Check sheet for the modelled part. Datum: model origin and axes. Units: mm. Face numbers are marked on the shaded views. Round coordinates to 2 decimals unless told otherwise and drop trailing zeros. Order: outer loops, then holes, each group sorted by start corner. A loop starts at its lowest first (then second) coordinate and runs counter-clockwise, first axis right, second up. Notation, with made-up numbers: (30.25, 41) -> (88.25, 41) arc R15 cw to (88.25, 68) -> close; hole circle Ø2 at (-22.5, 26). An arc over 180 degrees is marked (long way). Answer in a Markdown table with one row per item.
```python
from build123d import *

# Parameters (mm, degrees)
ESQUISSE1_W             = 24
ESQUISSE1_H             = 38
ESQUISSE1_W_2           = 10
ESQUISSE1_H_2           = 29.5
SHAPE_DEPTH             = 1.5
ESQUISSE2_R             = 1.2
VISHOLES_DEPTH          = 1.5
ESQUISSE3_R             = 1.8
LOCKERS_DEPTH           = 2
ESQUISSE4_R             = 2.2
SCREWHATREMOVER_DEPTH   = 0.5
ESQUISSE6_W             = 24
ESQUISSE6_H             = 14.5
RALLONGE_DEPTH          = 1.5
ESQUISSE7_W             = 24
ESQUISSE7_H             = 1.5
BOSS_EXTRU_2_DEPTH      = 8.5
ESQUISSE8_R             = 1.2
ENL_V_MAT_EXTRU_1_DEPTH = 10
ESQUISSE9_R             = 1.5
BOSS_EXTRU_3_DEPTH      = 5
NERVURE11_REACH         = 48.457
ESQUISSE12_WALL_W       = 106.934753954
ESQUISSE12_WALL_H       = 1


with BuildPart() as part:
    # Esquisse1 → Shape (new body)
    with BuildSketch(Plane(origin=(0, 0, 0), x_dir=(1, 0, 0), z_dir=(0, 1, 0))):
        Rectangle(ESQUISSE1_W, ESQUISSE1_H)
        with Locations((0, 2.75)):
            Rectangle(ESQUISSE1_W_2, ESQUISSE1_H_2, mode=Mode.SUBTRACT)
    extrude(amount=SHAPE_DEPTH)

    # Esquisse2 → VisHoles (cut)
    with BuildSketch(Plane(origin=(0, 1.5, 0), x_dir=(1, 0, 0), z_dir=(0, 1, 0))):
        with Locations(Location((10, -9, 0), (0, 0, 270))):
            Circle(ESQUISSE2_R)
    visholes = extrude(amount=-VISHOLES_DEPTH, mode=Mode.SUBTRACT)

    # Esquisse3 → Lockers (add)
    with BuildSketch(Plane(origin=(0, 1.5, 0), x_dir=(1, 0, 0), z_dir=(0, 1, 0))):
        with Locations(Location((10, 11, 0), (0, 0, 90))):
            Circle(ESQUISSE3_R)
    lockers = extrude(amount=LOCKERS_DEPTH)

    # Esquisse4 → ScrewHatRemover (cut)
    with BuildSketch(Plane(origin=(0, 0, 0), x_dir=(1, 0, 0), z_dir=(0, 1, 0))):
        with Locations((10, -9)):
            Circle(ESQUISSE4_R)
    screwhatremover = extrude(amount=SCREWHATREMOVER_DEPTH, mode=Mode.SUBTRACT)

    # Symétrie1: VisHoles, Lockers, ScrewHatRemover across plane
    add(visholes.mirror(Plane(origin=(0, 0, 0), x_dir=(0, 0, 1), z_dir=(1, 0, 0))), mode=Mode.SUBTRACT)
    add(lockers.mirror(Plane(origin=(0, 0, 0), x_dir=(0, 0, 1), z_dir=(1, 0, 0))))
    add(screwhatremover.mirror(Plane(origin=(0, 0, 0), x_dir=(0, 0, 1), z_dir=(1, 0, 0))), mode=Mode.SUBTRACT)

    # Esquisse6 → Rallonge (add)
    with BuildSketch(Plane.XZ):
        with Locations((0, 26.25)):
            Rectangle(ESQUISSE6_W, ESQUISSE6_H)
    extrude(amount=-RALLONGE_DEPTH)

    # Esquisse7 → Boss.-Extru.2 (add)
    with BuildSketch(Plane(origin=(0, 1.5, 0), x_dir=(1, 0, 0), z_dir=(0, 1, 0))):
        with Locations((0, -32.75)):
            Rectangle(ESQUISSE7_W, ESQUISSE7_H)
    extrude(amount=BOSS_EXTRU_2_DEPTH)

    # Esquisse8 → Enlèv. mat.-Extru.1 (cut)
    with BuildSketch(Plane.XY.offset(33.5)):
        with Locations((0, 5)):
            Circle(ESQUISSE8_R)
    extrude(amount=-ENL_V_MAT_EXTRU_1_DEPTH, mode=Mode.SUBTRACT)

    # Esquisse9 → Boss.-Extru.3 (add)
    with BuildSketch(Plane.XY.offset(33.5)):
        with Locations((5, 5)):
            Circle(ESQUISSE9_R)
        with Locations((-5, 5)):
            Circle(ESQUISSE9_R)
    extrude(amount=BOSS_EXTRU_3_DEPTH)

    # Esquisse12 wall → Nervure11 (add, up to next)
    with BuildSketch(Plane(origin=(-12, 5.75, 27.75), x_dir=(0, -0.707106781187, -0.707106781187), z_dir=(0, -0.707106781187, 0.707106781187)), mode=Mode.PRIVATE) as nervure11_sk1:
        with Locations((0, 0.5)):
            Rectangle(ESQUISSE12_WALL_W, ESQUISSE12_WALL_H)
    nervure11_tool1 = extrude(nervure11_sk1.sketch, amount=NERVURE11_REACH, mode=Mode.PRIVATE) - part.part
    nervure11 = nervure11_tool1.solids().sort_by_distance((-12, 5.75, 27.75))[0]
    add(nervure11)

    # Symétrie2: Nervure11 across plane
    add(nervure11.mirror(Plane(origin=(0, 0, 0), x_dir=(0, 0, 1), z_dir=(1, 0, 0))))


solid = part.part
```
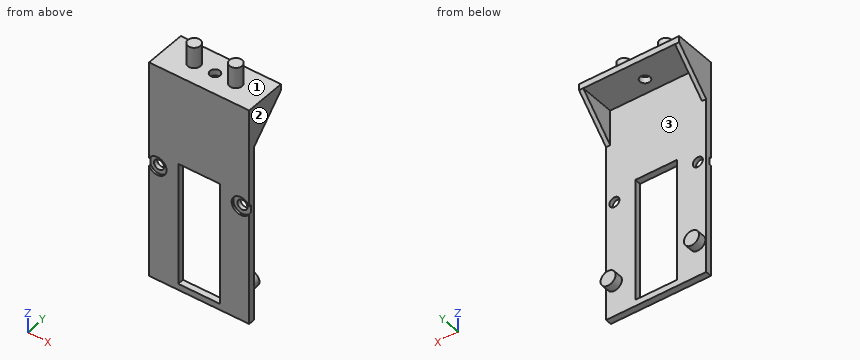
(1) Scan lines: probe 1 along X at (y, z) = (1.05, 9); probe 2 along Z at (x, y) = (-4.75, 0.5); probe 3 along Y at (x, z) = (0, 32.95). Record each from-to range of solid material in increasing order. Write a range as from..to.
Solutions:
| item | result |
|---|---|
| probe 1 | -12..-11.2, -8.8..-5, 5..8.8, 11.2..12 |
| probe 2 | -19..-17.5, 12..33.5 |
| probe 3 | 0..3.8, 6.2..10 |
(2) Section check A-A on x = -2.75. Record the boundary of the cut face in (y, z), plus the area to 4 significant figures.
Solutions:
| item | result |
|---|---|
| outline | (0, -19) -> (1.5, -19) -> (1.5, -17.5) -> (0, -17.5) -> close; (0, 12) -> (1.5, 12) -> (1.5, 32) -> (10, 32) -> (10, 33.5) -> (0, 33.5) -> close |
| area | 47.25 mm^2 |
(3) Draft check along Z on the marked faces 1, 2 and 3. Enter one of: pulls with the +Z half, pulls with the -Z half, needs draft (parallel to the pull), parting line crosses it, or undercut.
Solutions:
| item | result |
|---|---|
| face 1 | pulls with the +Z half |
| face 2 | needs draft |
| face 3 | undercut |
(4) Depth check by flat-ended pin: pin 1 Ø10 at (x, z) = (-9, 4.5) entering from +Y; pin 2 Ø1 at (x, y) = (-3.5, 2) entering from +Z; pin 3 Ø1.1 at (x, z) = (9.5, -10.5) entering from +Y; pin 4 Ø1.9 at (x, y) = (0, 5) entering from +Z. Enter the tip coordinate at first touch or a pass-through.
Solutions:
| item | result |
|---|---|
| pin 1 | y = 1.5 |
| pin 2 | z = 33.5 |
| pin 3 | y = 3.5 |
| pin 4 | through |
(5) Section check C-C on z = 9. Record the boundary of the cut face in (x, y), plus the area to 3 significant figures.
Solutions:
| item | result |
|---|---|
| outline | (-12, 0.5) -> (-11.2, 0.5) -> (-11.2, 1.5) -> (-12, 1.5) -> close; (-8.8, 0.5) -> (-7.8, 0.5) -> (-7.8, 0) -> (-5, 0) -> (-5, 1.5) -> (-8.8, 1.5) -> close; (5, 0) -> (7.8, 0) -> (7.8, 0.5) -> (8.8, 0.5) -> (8.8, 1.5) -> (5, 1.5) -> close; (11.2, 0.5) -> (12, 0.5) -> (12, 1.5) -> (11.2, 1.5) -> close |
| area | 12.0 mm^2 |
(6) Section check D-D on x = 0. Record the boundary of the cut face in (y, z), plus the area to 4 significant figures.
Solutions:
| item | result |
|---|---|
| outline | (0, -19) -> (1.5, -19) -> (1.5, -17.5) -> (0, -17.5) -> close; (0, 12) -> (1.5, 12) -> (1.5, 32) -> (3.8, 32) -> (3.8, 33.5) -> (0, 33.5) -> close; (6.2, 32) -> (10, 32) -> (10, 33.5) -> (6.2, 33.5) -> close |
| area | 43.65 mm^2 |
(7) Section check B-B on y = 5. Record the boundary of the cut face in (x, z).
Solutions:
| item | result |
|---|---|
| outline | (-12, 27) -> (-11, 27) -> (-11, 32) -> (-1.2, 32) -> (-1.2, 33.5) -> (-3.5, 33.5) -> (-3.5, 38.5) -> (-6.5, 38.5) -> (-6.5, 33.5) -> (-12, 33.5) -> close; (1.2, 32) -> (11, 32) -> (11, 27) -> (12, 27) -> (12, 33.5) -> (6.5, 33.5) -> (6.5, 38.5) -> (3.5, 38.5) -> (3.5, 33.5) -> (1.2, 33.5) -> close |
